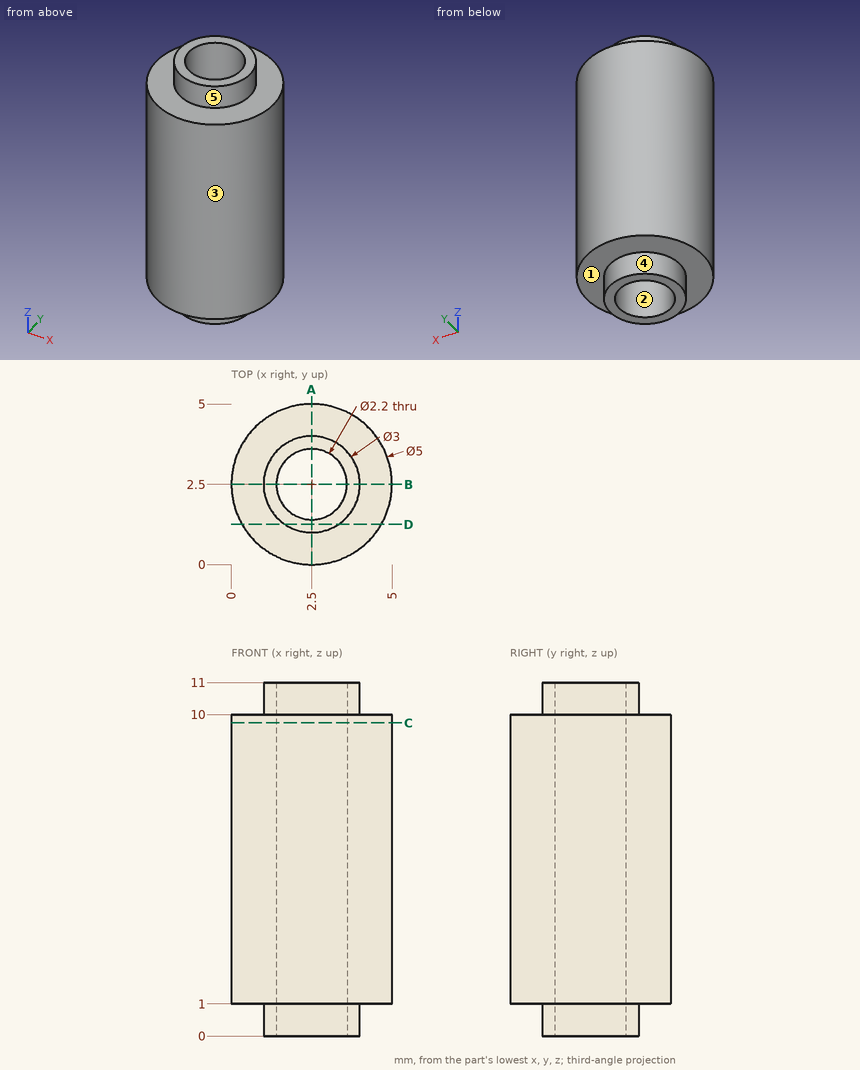
Job drawing, mm, ordinate dimensions from the low corner. One solid piece. A direction names the side the tool comes from. Coordinates: 2 decimals unless noted, no trailing zeros. Order: outer loops, then holes, each group sorted by start corner. A loop starts at its lowest first (then second) coordinate and runs counter-clockwise, first axis right, second up. Notation, with made-up numbers: (57.25, 49) - (63.25, 49) arc R19 ccw to (63.25, 70) - close; hole circle Ø7 at (-7.75, 8.5). An arc over 180 degrees is marked (long way). Write each question's results on one line, items separated by ' | '. Start each with the question number.
Item 1: Band-saw the part on C-C on z = 9.75. Write the cut outline in (x, y), and give its area (3 significant figures).
Item 2: Band-saw the part on A-A on x = 2.5. Write the cut outline in (y, z), and give its area (3 significant figures).
Item 3: Mould opens along Y. For the marked faces 1, 2 and 3 say: released by +Y, released by -Y, zero draft, split by the parting line, or undercut.
Item 4: Flat gauge pin, fed straight in: pin 1 (3 mm diameter, centred on x = 2.5, y = 2.5, fed in from +Z). Where does the tip first touch, or does it go through?
Item 5: Band-saw the part on D-D on y = 1.25. Write the cut outline in (x, z).
Item 6: Tool access for the marked faces 4 and 5: list every direction of +Z, -Z, +X, -X, +Y, -Y with a clear straight run to the whole face (end or side of a thin tool).
Item 7: Wall check: probe 1 along Y at (x, z) = (2.5, 4.5); probe 2 along Z at (x, y) = (3.95, 0.95); probe 3 along Y at (x, z) = (0.5, 9). Give the ranges that are in metal, low to high. Write a range as [from, to].
Numbers:
1) outline: circle Ø5 at (2.5, 2.5); hole circle Ø2.2 at (2.5, 2.5) | area: 15.8 mm^2
2) outline: (0, 1) - (1, 1) - (1, 0) - (1.4, 0) - (1.4, 11) - (1, 11) - (1, 10) - (0, 10) - close; (3.6, 0) - (4, 0) - (4, 1) - (5, 1) - (5, 10) - (4, 10) - (4, 11) - (3.6, 11) - close | area: 26.8 mm^2
3) face 1: zero draft | face 2: undercut | face 3: split by the parting line
4) pin 1: z = 11
5) outline: (0.33, 1) - (1.67, 1) - (1.67, 0) - (3.33, 0) - (3.33, 1) - (4.67, 1) - (4.67, 10) - (3.33, 10) - (3.33, 11) - (1.67, 11) - (1.67, 10) - (0.33, 10) - close
6) face 4: -Z | face 5: +Z
7) probe 1: [0, 1.4], [3.6, 5] | probe 2: [1, 10] | probe 3: [1, 4]
